from build123d import *

# Parameters (mm, degrees)
BOSS_EXTRUDE1_DEPTH     = 1260
SKETCH3_R               = 12.5
CUT_EXTRUDE1_DEPTH      = 8
CUT_EXTRUDE1_DEPTH_BACK = 8
FILLET1_R               = 5


with BuildPart() as part:
    # Sketch1 → Boss-Extrude1 (new body)
    with BuildSketch(Plane(origin=(0, 0, 0), x_dir=(1, 0, 0), z_dir=(0, 1, 0))):
        Polygon((15, 25), (15, 5.958548116), (8, 10), (8, -10), (15, -5.958548116), (15, -25), (-15, -25), (-15, -5.958548116), (-8, -10), (-8, 10), (-15, 5.958548116), (-15, 25), align=None)
    extrude(amount=BOSS_EXTRUDE1_DEPTH)

    # Sketch3 → Cut-Extrude1 (cut, two sides)
    with BuildSketch(Plane(origin=(0, 0, 0), x_dir=(0, 0, -1), z_dir=(1, 0, 0))) as cut_extrude1_sk:
        with Locations((0, 1210)):
            Circle(SKETCH3_R)
        with Locations((0, 1135)):
            Circle(SKETCH3_R)
        with Locations((0, 1060)):
            Circle(SKETCH3_R)
        with Locations((0, 985)):
            Circle(SKETCH3_R)
        with Locations((0, 910)):
            Circle(SKETCH3_R)
        with Locations((0, 835)):
            Circle(SKETCH3_R)
        with Locations((0, 760)):
            Circle(SKETCH3_R)
        with Locations((0, 685)):
            Circle(SKETCH3_R)
        with Locations((0, 610)):
            Circle(SKETCH3_R)
        with Locations((0, 535)):
            Circle(SKETCH3_R)
        with Locations((0, 460)):
            Circle(SKETCH3_R)
        with Locations((0, 385)):
            Circle(SKETCH3_R)
        with Locations((0, 310)):
            Circle(SKETCH3_R)
        with Locations((0, 235)):
            Circle(SKETCH3_R)
        with Locations((0, 160)):
            Circle(SKETCH3_R)
        with Locations((0, 85)):
            Circle(SKETCH3_R)
        with Locations((0, 10)):
            Circle(SKETCH3_R)
    extrude(amount=CUT_EXTRUDE1_DEPTH, mode=Mode.SUBTRACT)
    extrude(cut_extrude1_sk.sketch, amount=-CUT_EXTRUDE1_DEPTH_BACK, mode=Mode.SUBTRACT)

    # Fillet1
    fillet1_edges = [part.edges().sort_by_distance(p)[0] for p in [
        (15, 630, -25),
        (15, 630, 25),
        (-15, 630, 25),
        (-15, 630, -25),
    ]]
    fillet(fillet1_edges, radius=FILLET1_R)


solid = part.part
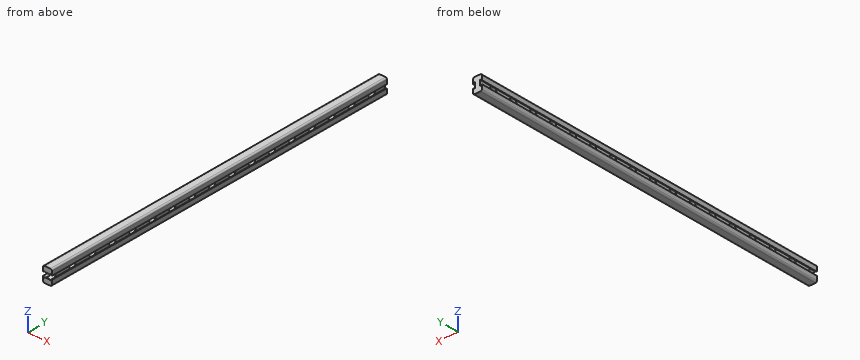
Source: CAD feature listing. Evaluate the final solid. Frame: model axes, mm. Coordinates: 2 decimals unless noted, no trailing zeros. Loops run counter-clockwise (first coordinate to the right, second up) from the corner with the lowest first, then second, coordinate; pieces in that order, holes last. Notation, with made-up numbers: (22.5, 17.25) -> (60.5, 17.25) arc R17 cw to (60.5, 36.25) -> close; hole circle Ø8 at (48.5, -38.75). An arc over 180 degrees is marked (long way). Answer in a Markdown table with one row per item. Add a question column.
Q1. Ray query, line 1 along X through (y, z) = (234, 10); line 2 along Z through (x, y) = (-3, 85); line 3 along X through (y, z) = (537, 9.5). Return the intervals inside material, ascending.
Q2. Contact query for a flat-ended pin moving along its axis: pin 1 Ø6 at (x, z) = (-3.5, 0.5) entering from -Y. Output: stop coordinate, or through.
Q3. Section A-A on y = 874. Return the cut outline in (x, z), and give its area (3 significant figures).
Computed values:
| question | item | result |
|---|---|---|
| 1 | line 1 | x = -15 to -8, 8 to 15 |
| 1 | line 2 | z = -25 to -12.5, 12.5 to 25 |
| 1 | line 3 | x = -15 to -8.87, 8.87 to 15 |
| 2 | pin 1 | stops at y = 22 |
| 3 | outline | (-15, -20) arc R5 ccw to (-10, -25) -> (10, -25) arc R5 ccw to (15, -20) -> (15, -5.96) -> (8, -10) -> (8, 10) -> (15, 5.96) -> (15, 20) arc R5 ccw to (10, 25) -> (-10, 25) arc R5 ccw to (-15, 20) -> (-15, 5.96) -> (-8, 10) -> (-8, -10) -> (-15, -5.96) -> close |
| 3 | area | 1,260 mm^2 |
